The model under review builds one solid part; all positions refer to its coordinate system, in mm. Coordinates: 2 decimals unless noted, no trailing zeros. Order: outer loops, then holes, each group sorted by start corner. A loop starts at its lowest first (then second) coordinate and runs counter-clockwise, first axis right, second up. Notation, with made-up numbers: (54.5, 47) -> (88.5, 47) arc R14 ccw to (88.5, 58) -> close; hole circle Ø3 at (88, 2). An arc over 180 degrees is marked (long way). Answer as CSV lines item,"result". Start each with the question number.
from build123d import *

# Parameters (mm, degrees)
SKETCH1_W           = 100
SKETCH1_H           = 1150
SKETCH1_W_2         = 68.25
SKETCH1_H_2         = 1118.25
BOSS_EXTRUDE1_DEPTH = 15.875
BOSS_EXTRUDE2_START = -15.875
BOSS_EXTRUDE2_DEPTH = 15.875
SKETCH5_W           = 195.875
SKETCH5_H           = 90
SKETCH5_W_2         = 164.125
SKETCH5_H_2         = 58.25
BOSS_EXTRUDE3_DEPTH = 7.9375
SKETCH6_W           = 15.875
SKETCH6_H           = 200
BOSS_EXTRUDE4_DEPTH = 15.875
CUT_EXTRUDE1_DEPTH  = 15.875
SKETCH8_W           = 50.625
SKETCH8_H           = 200.5
SKETCH8_W_2         = 18.875
SKETCH8_H_2         = 168.75
BOSS_EXTRUDE5_DEPTH = 15.875
BOSS_EXTRUDE6_DEPTH = 15.875


with BuildPart() as part:
    # Sketch1 → Boss-Extrude1 (new body)
    with BuildSketch(Plane(origin=(0, 0, 0), x_dir=(1, 0, 0), z_dir=(0, 1, 0))):
        Rectangle(SKETCH1_W, SKETCH1_H)
        Rectangle(SKETCH1_W_2, SKETCH1_H_2, mode=Mode.SUBTRACT)
    extrude(amount=BOSS_EXTRUDE1_DEPTH)

    # Sketch3 → Boss-Extrude2 (add)
    with BuildSketch(Plane(origin=(0, 15.875, 0), x_dir=(1, 0, 0), z_dir=(0, 1, 0)).offset(BOSS_EXTRUDE2_START)):
        Polygon((34.125, 400), (-130, 400), (-130, 220.59390888), (-130, -400), (34.125, -400), (50, -400), (50, -415.875), (-145.875, -415.875), (-145.875, 217.756753438), (-145.875, 415.875), (50, 415.875), (50, 400), align=None)
    extrude(amount=-BOSS_EXTRUDE2_DEPTH)

    # Sketch5 → Boss-Extrude3 (add, symmetric)
    with BuildSketch(Plane.XY):
        with Locations((-47.9375, 45)):
            Rectangle(SKETCH5_W, SKETCH5_H)
        with Locations((-47.9375, 45)):
            Rectangle(SKETCH5_W_2, SKETCH5_H_2, mode=Mode.SUBTRACT)
    extrude(amount=BOSS_EXTRUDE3_DEPTH, both=True)

    # Sketch6 → Boss-Extrude4 (add)
    with BuildSketch(Plane.XZ):
        with Locations((-26.1875, -459.125)):
            Rectangle(SKETCH6_W, SKETCH6_H)
        with Locations((26.1875, -459.125)):
            Rectangle(SKETCH6_W, SKETCH6_H)
    extrude(amount=-BOSS_EXTRUDE4_DEPTH)

    # Sketch7 → Cut-Extrude1 (cut)
    with BuildSketch(Plane.XZ):
        with BuildLine():
            Line((-23.1875, -374.125), (-23.1875, -514.125))
            ThreePointArc((-23.1875, -514.125), (-26.1875, -517.125), (-29.1875, -514.125))
            Line((-29.1875, -514.125), (-29.1875, -374.125))
            ThreePointArc((-29.1875, -374.125), (-26.1875, -371.125), (-23.1875, -374.125))
        make_face()
        with BuildLine():
            Line((29.1875, -374.125), (29.1875, -514.125))
            ThreePointArc((29.1875, -514.125), (26.1875, -517.125), (23.1875, -514.125))
            Line((23.1875, -514.125), (23.1875, -374.125))
            ThreePointArc((23.1875, -374.125), (26.1875, -371.125), (29.1875, -374.125))
        make_face()
    extrude(amount=-CUT_EXTRUDE1_DEPTH, mode=Mode.SUBTRACT)

    # Sketch8 → Boss-Extrude5 (add)
    with BuildSketch(Plane(origin=(0, 0, 0), x_dir=(1, 0, 0), z_dir=(0, 1, 0))):
        with Locations((-120.5625, -500.25)):
            Rectangle(SKETCH8_W, SKETCH8_H)
        with Locations((-120.5625, -500.25)):
            Rectangle(SKETCH8_W_2, SKETCH8_H_2, mode=Mode.SUBTRACT)
    extrude(amount=-BOSS_EXTRUDE5_DEPTH)

    # Sketch9 → Boss-Extrude6 (add)
    with BuildSketch(Plane(origin=(0, 0, 0), x_dir=(1, 0, 0), z_dir=(0, 1, 0))):
        Polygon((45.350320151, -404.649679849), (34.125, -415.875), (-145.875, -235.875), (-134.649679849, -224.649679849), align=None)
    boss_extrude6 = extrude(amount=-BOSS_EXTRUDE6_DEPTH)

    # Mirror1: Boss-Extrude6 across plane
    add(boss_extrude6.mirror(Plane.XY))


solid = part.part
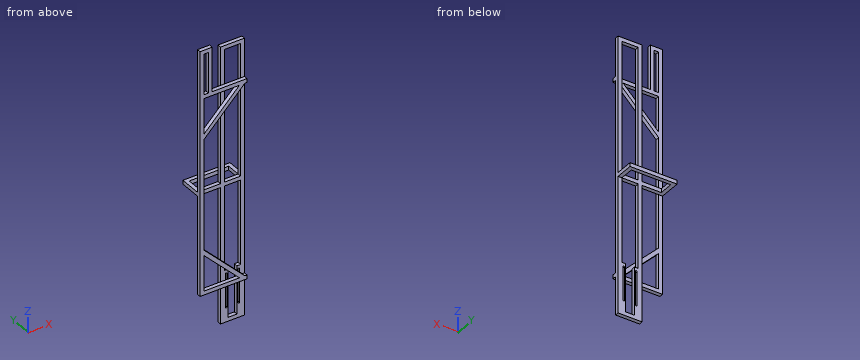
1) Insertion check: pin 1 Ø1.5 at (x, y) = (-78.5, -4) entering from -Z (3 decimals); pin 2 Ø5 at (y, z) = (7, -440) entering from -X; pin 3 Ø17.5 at (x, y) = (-28, -6.5) entering from -Z; pin 4 Ø8 at (x, y) = (-86, 9.5) entering from -Z. Each pin has a flat end and moves straight along its axis. Give the tip position at first contact, or say it passes through.
2) Consider section A-A (z = -193). Give the boundary of the cut face in (x, y) (3 decimals).
3) Consider section C-C (x = -2.5). Count the separate pieces of the cut face and the enclosed holes in it, plus the area to 3 significant figures.
4) Consider section B-B (y = 26). Give the boundary of the cut face in (x, z) (1 decimal).
5) Wall thickness on L1, parallel to Y at x = -35, z = 6.5 (3 decimals); L2, parallel to Z at x = -102, y = -6 (3 decimals); L3, parallel to X at y = 4, z = 289 (3 decimals): over which ranges is each line inside the solid? List them lowest first. Write a range as [from, to].
Result:
1,pin 1,"z = -415.875"
1,pin 2,"x = -50"
1,pin 3,"z = -575"
1,pin 4,"z = -7.94"
2,outline,"(-145.875, -15.875) -> (-130, -15.875) -> (-130, 0) -> (-145.875, 0) -> close; (-50, 0) -> (-34.125, 0) -> (-34.125, 15.875) -> (-50, 15.875) -> close; (34.125, 0) -> (50, 0) -> (50, 15.875) -> (34.125, 15.875) -> close"
3,separate pieces,"8"
3,enclosed holes,"0"
3,area,"2,220 mm2"
4,outline,"(-145.9, -7.9) -> (-130, -7.9) -> (-130, 7.9) -> (-145.9, 7.9) -> close; (34.1, -7.9) -> (50, -7.9) -> (50, 7.9) -> (34.1, 7.9) -> close"
5,L1,"[0, 15.875], [74.125, 90]"
5,L2,"[-415.875, -400], [-279.75, -257.299], [257.299, 279.75], [400, 600.5]"
5,L3,"[-50, -34.125], [34.125, 50]"
